Can you work these out from the model? Positions are in its coordinate system, mm. A direction names the side the tool comes from. Give positions to 0.01 mm unless a question says otherwise; leave off trailing zeros. Order: outer loops, then holes, each group sorted by start corner. A loop starts at its lowest first (then second) coordinate and runs counter-clockwise, first axis right, second up.
Item 1: I'm going to push flat-ended pins straight in: pin 1 Ø2 at (y, z) = (2, 40) entering from -X; pin 2 Ø3.5 at (x, y) = (35.5, -2.5) entering from -Z; pin 3 Ø4 at (y, z) = (2, -77) entering from -X. Where does each tip first touch, or does it pass through?
Item 2: I want a section at B-B, the plane x = -64.5. Write out the boundary of the cut face in (y, z), then the cut area to 3 significant figures.
Item 3: Which directions (+Z, -Z, +X, -X, +Y, -Y) give clear straight access to the entire face, cutting with the end or side of a thin tool? Please do faces 1 (the flat face through (-64.186, -0.084, 58.849)), 2 (the flat face through (-2, 6, -24)).
Item 4: I want a section at C-C, the plane z = 101.5. Write out the boundary of the cut face in (x, y).
Item 5: I want a section at A-A, the plane y = -3.25. Write out the boundary of the cut face in (x, z).
Item 6: If we mould it in two halves opening along Z, with no side actions, what happens to faces 3 (the flat face through (-63.792, -0.084, -57.816)), 4 (the flat face through (31, 0, -32.5)), 5 (the flat face through (31, 0, 32.5))? For each: +Z half, -Z half, draft (parallel to the pull), parting line (faces both ways), or undercut.
Item 7: If I drill on line 1 along Z through (x, y) = (0, 2); line 2 along X through (y, z) = (-2, 99); line 3 along Z through (x, y) = (46, -2.75), over which ranges is the centre line in solid material (lowest first)?
Item 8: I want a section at D-D, the plane x = 0. Write out the boundary of the cut face in (y, z), then the cut area to 3 significant figures.
```python
from build123d import *

# Parameters (mm, degrees)
F1_DEPTH = 6
F2_R     = 2.5
F3_DEPTH = 12.001


# Not quite as in the source:
# - a feature names something its author has since deleted; it is built from what else it names


with BuildPart() as f1:
    # F0 (on Front) → F1 (new body, symmetric)
    with BuildSketch(Plane.XZ):
        Polygon((43.524, -32.5), (121.5, -20), (121.5, 20), (43.524, 32.5), (25, 32.5), (18.7638837487, 32.5), (15.645825623, 37.9006350946), (6.383825623, 53.9428896743), (-43.4294919243, 115.2220865598), (-78.0705080757, 95.2220865598), (-49.907825623, 21.4428896743), (-40.645825623, 5.4006350946), (-37.5277674973, 0), (-40.645825623, -5.4006350946), (-49.907825623, -21.4428896743), (-78.0705080757, -95.2220865598), (-43.4294919243, -115.2220865598), (6.383825623, -53.9428896743), (15.645825623, -37.9006350946), (18.7638837487, -32.5), (25, -32.5), align=None)
    extrude(amount=F1_DEPTH, both=True)

    # F2 (on face) → F3 (cut, through all)
    with BuildSketch(Plane.XZ.offset(6)):
        Circle(F2_R)
    extrude(amount=-F3_DEPTH, mode=Mode.SUBTRACT)


solid = f1.part
```
Results list:
1. pin 1: stops at x = -57.37
1. pin 2: stops at z = -32.5
1. pin 3: stops at x = -71.88
2. outline: (-6, -103.06) - (6, -103.06) - (6, -59.67) - (-6, -59.67) - close; (-6, 59.67) - (6, 59.67) - (6, 103.06) - (-6, 103.06) - close
2. area: 1,040 mm2
3. face 1: -X, +Y, -Y
3. face 2: +Z, -Z, +X, -X, +Y
4. outline: (-67.2, -6) - (-32.27, -6) - (-32.27, 6) - (-67.2, 6) - close
5. outline: (-78.07, -95.22) - (-43.43, -115.22) - (6.38, -53.94) - (18.76, -32.5) - (43.52, -32.5) - (121.5, -20) - (121.5, 20) - (43.52, 32.5) - (18.76, 32.5) - (6.38, 53.94) - (-43.43, 115.22) - (-78.07, 95.22) - (-49.91, 21.44) - (-37.53, 0) - (-49.91, -21.44) - close; hole circle Ø5 at (0, 0)
6. face 3: undercut
6. face 4: -Z half
6. face 5: +Z half
7. line 1: z = -61.8 to -2.5, 2.5 to 61.8
7. line 2: x = -71.53 to -30.24
7. line 3: z = -32.1 to 32.1
8. outline: (-6, -61.8) - (6, -61.8) - (6, -2.5) - (-6, -2.5) - close; (-6, 2.5) - (6, 2.5) - (6, 61.8) - (-6, 61.8) - close
8. area: 1,420 mm2
